```python
from build123d import *

# Parameters (mm, degrees)
F0_R      = 141.361555
F1_DEPTH  = 201.93
F3_W      = 134.041112
F3_H      = 116.143879
F4_DEPTH  = 112.395
F5_R      = 25.4
F7_R      = 23.556914
F8_DEPTH  = 25.4
F9_R      = 70.475259
F10_DEPTH = 120.65


with BuildPart() as f1:
    # F0 (on Top) → F1 (new body)
    with BuildSketch(Plane.XY):
        Circle(F0_R)
    extrude(amount=F1_DEPTH)

    # F3 (on face) → F4 (join)
    with BuildSketch(Plane.XY.offset(201.93)):
        with Locations((9.092184, 11.829982)):
            Rectangle(F3_W, F3_H)
    extrude(amount=F4_DEPTH)

    # F5
    f5_edges = [f1.edges().sort_by_distance(p)[0] for p in [
        (-141.361555, 0, 201.93),
    ]]
    fillet(f5_edges, radius=F5_R)

    # F7 (on face) → F8 (join)
    with BuildSketch(Plane.XY.offset(314.325)):
        with Locations((29.327184, 28.160922)):
            Circle(F7_R)
    extrude(amount=F8_DEPTH)

    # F9 (on face) → F10 (join)
    with BuildSketch(Plane.XY.offset(314.325)):
        with Locations((78.396186, -45.443591)):
            Circle(F9_R)
    extrude(amount=F10_DEPTH)


solid = f1.part
```
The model under review builds one solid part; all positions refer to its coordinate system, in mm. A direction names the side the tool comes from. Round coordinates to 2 decimals unless told otherwise and drop trailing zeros. Write each loop counter-clockwise with the first axis right and the second up, starting at its lowest first coordinate (ties: lowest second). Pieces come first, ordered by that corner, then holes.
(1) Wall thickness on L1, parallel to Z at x = 46.5, y = -60 (3 decimals); L2, parallel to Z at x = 4, y = 59 (3 decimals); L3, parallel to Z at x = -105.5, y = -15.5: over which ranges is each line inside the solid? List them lowest first.
(2) Insertion check: pin 1 (1.5 mm diameter, centred on x = -78, z = 115, fed in from +Y); pin 2 (12 mm diameter, centred on y = -57.5, z = 155, fed in from -X); pin 3 (2 mm diameter, centred on x = 29, z = 381, fed in from -Y). Each pin has a flat end and moves straight along its axis. Give the tip position at first contact, or say it passes through.
(3) We need section C-C on z = 239. Give the boundary of the cut face in (x, y).
(4) Machinability: for faces 4 (the flat face through (8, -46.242, 257)), 5 (the flat face through (76.113, 11, 257)), 6 (the flat face through (-57.928, 11, 257)), 7 (the flat face through (-7, 26, 314.325)), which of the approach directions +Z, -Z, +X, -X, +Y, -Y give a long, thin tool a straight path to every point of the face, cutting with its end or side? Answer none if there is none.
(5) We need section A-A on x = 0. Give the boundary of the cut face in (y, z) (3 decimals), and give its area (3 significant figures).
(6) Mouldability with a two-part tool opening along Y and no side actions: class faces 1 (the cylindrical face through (16.96, 48.21, 326.85)), 2 (the flat face through (-2, 2, 0)), 3 (the cylindrical face through (-141.225, 6.215, 87.029)) as +Y half, -Y half, draft (parallel to the pull), parting line (faces both ways), or undercut.
(7) We need section B-B on z = 96. Give the boundary of the cut face in (x, y).
Findings below:
1. L1: z = 0 to 201.93, 314.325 to 434.975
1. L2: z = 0 to 314.325
1. L3: z = 0 to 201.93
2. pin 1: stops at y = 118.39
2. pin 2: stops at x = -131.65
2. pin 3: stops at y = -96.67
3. outline: (-57.93, -46.24) - (76.11, -46.24) - (76.11, 69.9) - (-57.93, 69.9) - close
4. face 4: +X, -X, -Y
4. face 5: +X, +Y, -Y
4. face 6: +Z, -X, +Y, -Y
4. face 7: +Z
5. outline: (-141.362, 0) - (141.362, 0) - (141.362, 176.53) arc R25.4 ccw to (115.962, 201.93) - (69.902, 201.93) - (69.902, 314.325) - (-46.242, 314.325) - (-46.242, 201.93) - (-115.962, 201.93) arc R25.4 ccw to (-141.362, 176.53) - close
5. area: 69,900 mm2
6. face 1: undercut
6. face 2: draft
6. face 3: parting line
7. outline: circle Ø282.72 at (0, 0)
